Verification items for the finished model (mm, model axes). Face numbers are marked on the shaded views. Give positions to 0.01 mm unless a question says otherwise; leave off trailing zeros. Order: outer loops, then holes, each group sorted by start corner. A loop starts at its lowest first (then second) coordinate and runs counter-clockwise, first axis right, second up.
(1) Sectioned sample at A-A on z = 5. Record the cut outline in (x, y), plus the area to 3 significant figures.
(2) Mould release check, pull along X, two halves, no side actions. Record for the marked faces 1, 2 and 3: pulls with the +X half, pulls with the -X half, needs draft (parallel to the pull), parting line crosses it, or undercut.
(3) Gauge pin test, flat ends, axial feed: pin 1 (4 mm diameter, centred on x = -3, y = -13.5, fed in from -Z); pin 2 (8 mm diameter, centred on y = 17.5, z = 3.5, fed in from -X); pin 3 (3 mm diameter, centred on y = 19.5, z = -8.5, fed in from +X). Record the tip position at first contact, or that the pin passes through.
(4) Sectioned sample at B-B on x = 0. Record the cut outline in (y, z), plus the area to 3 significant figures.
(5) Scan lines: L1, parallel to Y at x = 0, z = -6.75; L2, parallel to Z at x = -14, y = -4; L3, parallel to Y at x = 9, z = -0.25. Record each from-to range of solid material in increasing order.
```python
from build123d import *

# Parameters (mm, degrees)
F0_R     = 25.4
F1_DEPTH = 12.7
F2_T     = -2.54
F3_R     = 2.54


with BuildPart() as f1:
    # F0 (on Top) → F1 (new body, symmetric)
    with BuildSketch(Plane.XY):
        Circle(F0_R)
    extrude(amount=F1_DEPTH, both=True)

    # F2
    f2_openings = [f1.faces().sort_by_distance(p)[0] for p in [
        (0, 0, -12.7),
    ]]
    offset(amount=F2_T, openings=f2_openings)

    # F3
    f3_edges = [f1.edges().sort_by_distance(p)[0] for p in [
        (-25.4, 0, 12.7),
    ]]
    fillet(f3_edges, radius=F3_R)


solid = f1.part
```
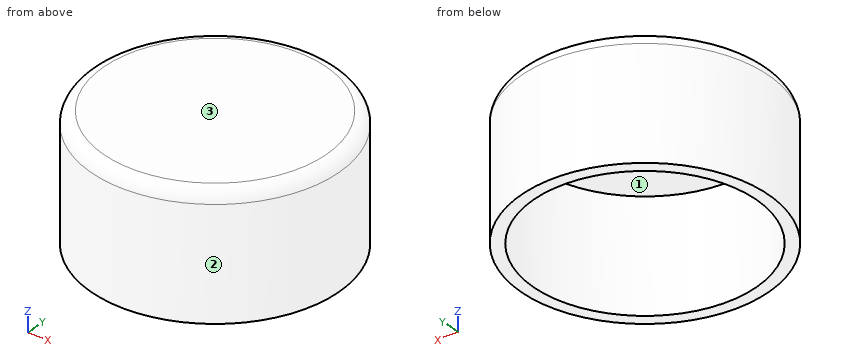
Ans:
1. outline: circle Ø50.8 at (0, 0); hole circle Ø45.72 at (0, 0)
1. area: 385 mm2
2. face 1: undercut
2. face 2: parting line crosses it
2. face 3: needs draft
3. pin 1: stops at z = 10.16
3. pin 2: stops at x = -21.52
3. pin 3: stops at x = 17.92
4. outline: (-25.4, -12.7) - (-22.86, -12.7) - (-22.86, 10.16) - (22.86, 10.16) - (22.86, -12.7) - (25.4, -12.7) - (25.4, 10.16) arc R2.54 ccw to (22.86, 12.7) - (-22.86, 12.7) arc R2.54 ccw to (-25.4, 10.16) - close
4. area: 242 mm2
5. L1: y = -25.4 to -22.86, 22.86 to 25.4
5. L2: z = 10.16 to 12.7
5. L3: y = -23.75 to -21.01, 21.01 to 23.75
